Here's the drawing with two shaded views (mm, measured from the low corner). I have some questions. A direction names the side the tool comes from. Round coordinates to 2 decimals unless told otherwise and drop trailing zeros. Loops run counter-clockwise (first coordinate to the right, second up) from the corner with the lowest first, then second, coordinate; pieces in that order, holes last.
(1) Which directions (+Z, -Z, +X, -X, +Y, -Y) give clear straight access to the entire face, cutting with the end or side of a thin tool? Please do the marked faces 1 and 2.
(2) I want a section at D-D on z = 4.3. Write out the boundary of the cut face in (x, y).
(3) If I drill on line 1 along X through (y, z) = (3.1, 2.5); line 2 along X through (y, z) = (2.5, 2); line 3 along X through (y, z) = (0.9, 4.1), over which ranges is the centre line in solid material (lowest first)?
(4) Thinking about a two-plate mould opening in X: for the marked faces 3, 4 and 5, which applies, released by +X, released by -X, zero draft, split by the parting line, or undercut?
(5) I want a section at C-C on x = 15.25. Write out the boundary of the cut face in (y, z).
(6) I want a section at A-A on z = 2.5. Write out the boundary of the cut face in (x, y).
(7) Will this pin go through, and if not, where does the flat tip stop? pin 1 Ø1 at (x, z) = (12, 2) entering from -Y.
(8) I want a section at B-B on y = 0.7. Write out the boundary of the cut face in (x, z), plus the area to 3 significant figures.
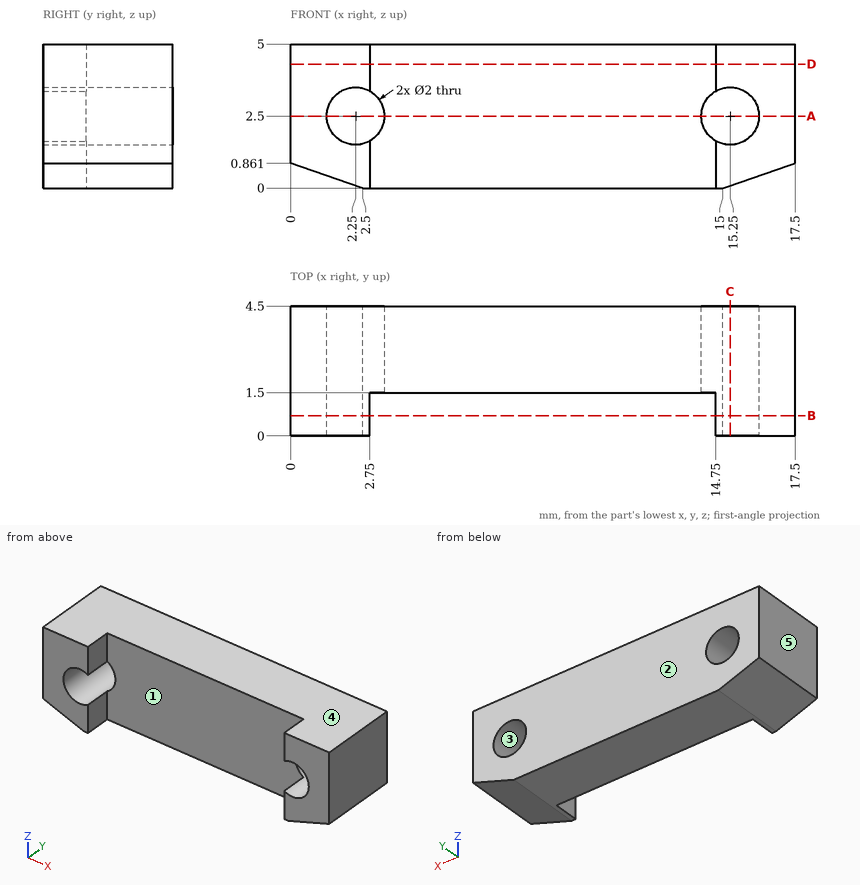
Filled sheet:
1. face 1: +Z, -Z, -Y
1. face 2: +Z, -Z, +X, -X, +Y
2. outline: (0, 0) - (2.75, 0) - (2.75, 1.5) - (14.75, 1.5) - (14.75, 0) - (17.5, 0) - (17.5, 4.5) - (0, 4.5) - close
3. line 1: x = 0 to 1.25, 3.25 to 14.25, 16.25 to 17.5
3. line 2: x = 0 to 1.38, 3.12 to 14.38, 16.12 to 17.5
3. line 3: x = 0 to 2.75, 14.75 to 17.5
4. face 3: undercut
4. face 4: zero draft
4. face 5: released by -X
5. outline: (0, 0.09) - (4.5, 0.09) - (4.5, 1.5) - (0, 1.5) - close; (0, 3.5) - (4.5, 3.5) - (4.5, 5) - (0, 5) - close
6. outline: (0, 0) - (1.25, 0) - (1.25, 4.5) - (0, 4.5) - close; (3.25, 1.5) - (14.25, 1.5) - (14.25, 4.5) - (3.25, 4.5) - close; (16.25, 0) - (17.5, 0) - (17.5, 4.5) - (16.25, 4.5) - close
7. pin 1: stops at y = 1.5
8. outline: (0, 0.86) - (2.5, 0) - (2.75, 0) - (2.75, 1.63) arc R1 cw (long way) to (2.75, 3.37) - (2.75, 5) - (0, 5) - close; (14.75, 0) - (15, 0) - (17.5, 0.86) - (17.5, 5) - (14.75, 5) - (14.75, 3.37) arc R1 cw (long way) to (14.75, 1.63) - close
8. area: 20.3 mm2
